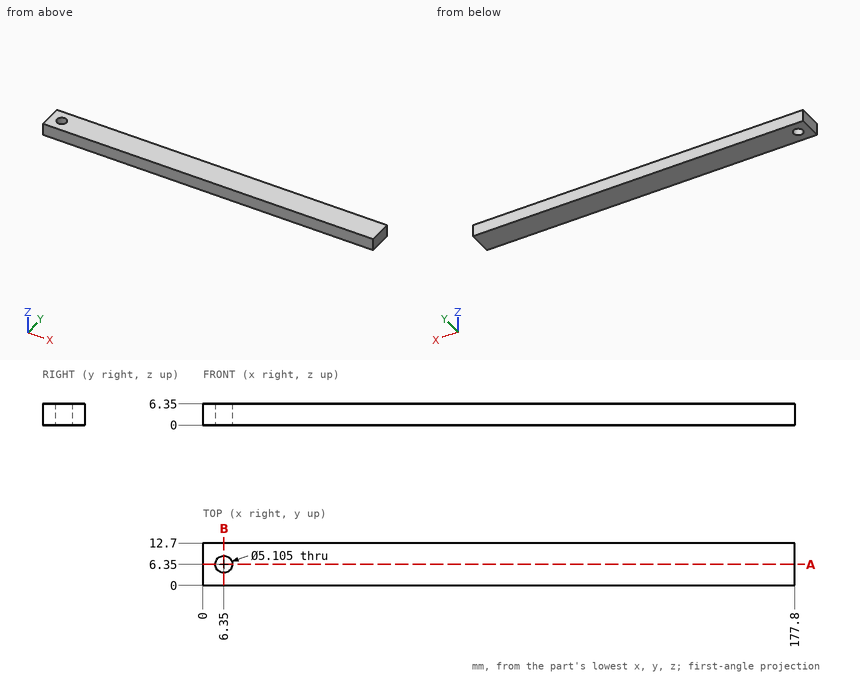
Geometry check sheet. Reference: drawing and pictorial views, mm from the part's lowest x, y, z. Round coordinates to 2 decimals unless told otherwise and drop trailing zeros. Loops run counter-clockwise (first coordinate to the right, second up) from the corner with the lowest first, then second, coordinate; pieces in that order, holes last. Notation, with made-up numbers: (66.25, -31.75) - (100.25, -31.75) arc R14 ccw to (100.25, -24.75) - close; hole circle Ø10 at (38, 40.25). An arc over 180 degrees is marked (long way). Write item = value, one per line. Start each with the question number.
Q1. Depth check by flat-ended pin: P1, Ø2, axis at y = 6.5, z = 3.5, coming from the -X side. Enter the tip coordinate at first touch or a pass-through.
Q2. Thickness scan on L1, parallel to X at y = 6.35, z = 4; L2, parallel to X at y = 5.5, z = 0.5. Record the ranges inside material, lowest first.
Q3. Section check A-A (y = 6.35). Record the boundary of the cut face in (x, z).
Q4. Section check B-B (x = 6.35). Record the boundary of the cut face in (y, z).
Derived:
q1.P1 = 0
q2.L1 = 0 to 3.8, 8.9 to 177.8
q2.L2 = 0 to 3.94, 8.76 to 177.8
q3.outline = (0, 0) - (3.8, 0) - (3.8, 6.35) - (0, 6.35) - close; (8.9, 0) - (177.8, 0) - (177.8, 6.35) - (8.9, 6.35) - close
q4.outline = (0, 0) - (3.8, 0) - (3.8, 6.35) - (0, 6.35) - close; (8.9, 0) - (12.7, 0) - (12.7, 6.35) - (8.9, 6.35) - close
